from build123d import *

# Parameters (mm, degrees)
ESBO_O3_W                = 7
ESBO_O3_H                = 12
ESBO_O3_R                = 1.75
RESSALTO_EXTRUS_O2_DEPTH = 2.7
ESBO_O4_W                = 7
ESBO_O4_H                = 12
ESBO_O4_R                = 1.75
RESSALTO_EXTRUS_O3_DEPTH = 2.1
ESBO_O5_W                = 2.1
ESBO_O5_H                = 12
RESSALTO_EXTRUS_O4_DEPTH = 5
RESSALTO_EXTRUS_O5_DEPTH = 3
ESBO_O7_W                = 4.8
ESBO_O7_H                = 15
RESSALTO_EXTRUS_O6_DEPTH = 3
ESBO_O8_R                = 2.9
CORTE_EXTRUS_O1_DEPTH    = 3
FILETE1_R                = 5.5
RESSALTO_EXTRUS_O7_DEPTH = 1.5
CORTE_EXTRUS_O4_DEPTH    = 6.3
CORTE_EXTRUS_O5_DEPTH    = 6.3
RESSALTO_EXTRUS_O8_DEPTH = 0.3
CORTE_EXTRUS_O6_DEPTH    = 0.3
ESBO_O17_R               = 2.9
CORTE_EXTRUS_O7_DEPTH    = 0.3


with BuildPart() as part:
    # Esboço3 → Ressalto-extrusão2 (new body)
    with BuildSketch(Plane.XY):
        with Locations((-3.5, 6)):
            Rectangle(ESBO_O3_W, ESBO_O3_H)
        with Locations((-2.5, 2.5)):
            Circle(ESBO_O3_R, mode=Mode.SUBTRACT)
    extrude(amount=RESSALTO_EXTRUS_O2_DEPTH)

    # Esboço4 → Ressalto-extrusão3 (add)
    with BuildSketch(Plane.XY.offset(2.7)):
        with Locations((-3.5, 6)):
            Rectangle(ESBO_O4_W, ESBO_O4_H)
        with Locations((-2.5, 2.5)):
            Circle(ESBO_O4_R, mode=Mode.SUBTRACT)
    extrude(amount=RESSALTO_EXTRUS_O3_DEPTH)

    # Esboço5 → Ressalto-extrusão4 (add)
    with BuildSketch(Plane.ZY.offset(7)):
        with Locations((3.75, 6)):
            Rectangle(ESBO_O5_W, ESBO_O5_H)
    extrude(amount=RESSALTO_EXTRUS_O4_DEPTH)

    # Esboço6 → Ressalto-extrusão5 (add)
    with BuildSketch(Plane.XZ):
        Polygon((-7, 0), (0, 0), (0, 4.8), (-12, 4.8), (-12, 2.7), (-7, 2.7), align=None)
    extrude(amount=RESSALTO_EXTRUS_O5_DEPTH)

    # Esboço7 → Ressalto-extrusão6 (add)
    with BuildSketch(Plane(origin=(0, 0, 0), x_dir=(0, 0, -1), z_dir=(1, 0, 0))):
        with Locations((-2.4, 4.5)):
            Rectangle(ESBO_O7_W, ESBO_O7_H)
    extrude(amount=RESSALTO_EXTRUS_O6_DEPTH)

    # Esboço8 → Corte-extrusão1 (cut)
    with BuildSketch(Plane.XY.offset(4.8)):
        with Locations((-2.5, 2.5)):
            Circle(ESBO_O8_R)
    extrude(amount=-CORTE_EXTRUS_O1_DEPTH, mode=Mode.SUBTRACT)

    # Filete1
    filete1_edges = [part.edges().sort_by_distance(p)[0] for p in [
        (3, -3, 2.4),
    ]]
    fillet(filete1_edges, radius=FILETE1_R)

    # Esboço10 → Ressalto-extrusão7 (add)
    with BuildSketch(Plane(origin=(0, 0, 0), x_dir=(-1, 0, 0), z_dir=(0, 0, -1))):
        with BuildLine():
            Line((7, 0), (0, 0))
            Line((0, 0), (0, 12))
            Line((0, 12), (-3, 12))
            Line((-3, 12), (-3, 2.5))
            ThreePointArc((-3, 2.5), (-1.389087297, -1.389087297), (2.5, -3))
            Line((2.5, -3), (7, -3))
            Line((7, -3), (7, 0))
        make_face()
    extrude(amount=RESSALTO_EXTRUS_O7_DEPTH)

    # Esboço14 → Corte-extrusão4 (cut)
    with BuildSketch(Plane.XY.offset(4.8)):
        with BuildLine():
            Line((-12, 12), (-12, 6.5))
            ThreePointArc((-12, 6.5), (-10.389087297, 10.389087297), (-6.5, 12))
            Line((-6.5, 12), (-12, 12))
        make_face()
        with BuildLine():
            ThreePointArc((-2.5, 12), (1.389087297, 10.389087297), (3, 6.5))
            Line((3, 6.5), (3, 12))
            Line((3, 12), (-2.5, 12))
        make_face()
    extrude(amount=-CORTE_EXTRUS_O4_DEPTH, mode=Mode.SUBTRACT)

    # Esboço13 → Corte-extrusão5 (cut)
    with BuildSketch(Plane.XY.offset(4.8)):
        with BuildLine():
            Line((-12, -3), (-6.5, -3))
            ThreePointArc((-6.5, -3), (-10.389087297, -1.389087297), (-12, 2.5))
            Line((-12, 2.5), (-12, -3))
        make_face()
    extrude(amount=-CORTE_EXTRUS_O5_DEPTH, mode=Mode.SUBTRACT)

    # Esboço15 → Ressalto-extrusão8 (add)
    with BuildSketch(Plane(origin=(0, 0, -1.5), x_dir=(-1, 0, 0), z_dir=(0, 0, -1))):
        with BuildLine():
            Line((2.5, -3), (6.5, -3))
            ThreePointArc((6.5, -3), (6.750259203, -2.994303444), (7, -2.977225575))
            Line((7, -2.977225575), (7, 0))
            Line((7, 0), (0, 0))
            Line((0, 0), (0, 11.398979486))
            ThreePointArc((0, 11.398979486), (-2.19041576, 9.372281323), (-3, 6.5))
            Line((-3, 6.5), (-3, 2.5))
            ThreePointArc((-3, 2.5), (-1.389087297, -1.389087297), (2.5, -3))
        make_face()
    extrude(amount=RESSALTO_EXTRUS_O8_DEPTH)

    # Esboço16 → Corte-extrusão6 (cut)
    with BuildSketch(Plane.XY.offset(4.8)):
        with BuildLine():
            Line((-12, 6.5), (-12, 2.5))
            ThreePointArc((-12, 2.5), (-10.389087297, -1.389087297), (-6.5, -3))
            Line((-6.5, -3), (-2.5, -3))
            ThreePointArc((-2.5, -3), (1.389087297, -1.389087297), (3, 2.5))
            Line((3, 2.5), (3, 6.5))
            ThreePointArc((3, 6.5), (1.389087297, 10.389087297), (-2.5, 12))
            Line((-2.5, 12), (-6.5, 12))
            ThreePointArc((-6.5, 12), (-10.389087297, 10.389087297), (-12, 6.5))
        make_face()
    extrude(amount=-CORTE_EXTRUS_O6_DEPTH, mode=Mode.SUBTRACT)

    # Esboço17 → Corte-extrusão7 (cut)
    with BuildSketch(Plane.XY.offset(1.8)):
        with Locations((-2.5, 2.5)):
            Circle(ESBO_O17_R)
    extrude(amount=-CORTE_EXTRUS_O7_DEPTH, mode=Mode.SUBTRACT)


solid = part.part
Can you work these out from the model? Positions are in its coordinate system, mm. A direction names the side the tool comes from. Coordinates: 2 decimals unless noted, no trailing zeros. Write each loop counter-clockwise with the first axis right and the second up, starting at its lowest first coordinate (ties: lowest second). Pieces come first, ordered by that corner, then holes. Notation, with made-up numbers: (-21, -9) - (13, -9) arc R21 ccw to (13, 9) - close; hole circle Ø8 at (-18.75, 5.25). An arc over 180 degrees is marked (long way). Return JSON: item names as keys, results as strings. Group by question number.
Item 1: Please list where these lines run through material, in increasing order: probe 1 along Y at (x, z) = (-2.5, 0.5); probe 2 along X at (y, z) = (2.5, 0.5); probe 3 along Y at (x, z) = (-2.5, 3.9).
Item 2: If we section it at C-C (y = 6): Write out the boundary of the cut face in (x, z), then the cut area to 3 significant figures.
Item 3: If we section it at B-B (x = -2.25): Write out the boundary of the cut face in (y, z).
Item 4: Which directions (+Z, -Z, +X, -X, +Y, -Y) give clear straight access to the entire face, cutting with the end or side of a thin tool? Please do faces 5 (the face through (-10, 5, 2.7)), 6 (the face through (-4, 6, 0)), 7 (the face through (-0.941, 4.945, 3.021)).
Item 5: I'm going to push flat-ended pins straight in: pin 1 Ø1.4 at (x, z) = (-4, -1) entering from +Y; pin 2 Ø5.5 at (x, y) = (-10, 4) entering from -Z; pin 3 Ø5.5 at (x, y) = (-2.5, 2.5) entering from -Z; pin 4 Ø3 at (x, y) = (-5, 7.5) entering from -Z. Where does each tip first touch, or does it pass through?
Item 6: If we section it at A-A (z = 2): Write out the boundary of the cut face in (x, y).
Item 7: We'd pull the mould along X, two halves only. Please class faces 1 (the face through (-4, 0, -1)), 2 (the face through (-10.43, 10.35, 3.28)), 3 (the face through (-1, 1, 1.5)), 4 (the face through (1.43, -1.35, 1.39)): pulls with the +X half, pulls with the -X half, needs draft (parallel to the pull), parting line crosses it, or undercut.
Item 8: If we section it at D-D (z = -0.25): Write out the boundary of the cut face in (x, y), then the cut area to 3 significant figures.
Return value:
{
 "1": {"probe 1": "y = -3 to 0.75, 4.25 to 12", "probe 2": "x = -7 to -4.25, -0.75 to 3", "probe 3": "y = -3 to -0.4, 5.4 to 12"},
 "2": {"outline": "(-12, 2.7) - (-7, 2.7) - (-7, 0) - (0, 0) - (0, -1.8) - (3, -1.8) - (3, 4.5) - (-12, 4.5) - close", "area": "59.4 mm^2"},
 "3": {"outline": "(-2.99, -1.8) - (0, -1.8) - (0, 0) - (0.77, 0) - (0.77, 1.5) - (-0.39, 1.5) - (-0.39, 4.5) - (-2.99, 4.5) - close; (4.23, 0) - (11.99, 0) - (11.99, 4.5) - (5.39, 4.5) - (5.39, 1.5) - (4.23, 1.5) - close"},
 "4": {"face 5": "-Z, -X, +Y, -Y", "face 6": "-Z, -X, +Y", "face 7": "+Z"},
 "5": {"pin 1": "stops at y = 0", "pin 2": "stops at z = 2.7", "pin 3": "stops at z = -1.8", "pin 4": "stops at z = 0"},
 "6": {"outline": "(-7, -2.98) arc R5.5 ccw to (-6.5, -3) - (-2.5, -3) arc R5.5 ccw to (3, 2.5) - (3, 6.5) arc R5.5 ccw to (-2.5, 12) - (-6.5, 12) arc R5.5 ccw to (-7, 11.98) - close; hole circle Ø5.8 at (-2.5, 2.5)"},
 "7": {"face 1": "needs draft", "face 2": "pulls with the -X half", "face 3": "undercut", "face 4": "pulls with the +X half"},
 "8": {"outline": "(-7, -2.98) arc R5.5 ccw to (-6.5, -3) - (-2.5, -3) arc R5.5 ccw to (3, 2.5) - (3, 6.5) arc R5.5 ccw to (0, 11.4) - (0, 0) - (-7, 0) - close", "area": "53.5 mm^2"}
}
